```python
from build123d import *

# Parameters (mm, degrees)
SCHIZZO1_R                   = 20
SCHIZZO1_R_2                 = 1.6
ESTRUSIONE_ESTRUSIONE1_DEPTH = 10
TAGLIO_ESTRUSIONE1_DEPTH     = 3
RACCORDO1_R                  = 2
SCHIZZO3_R                   = 5
SCHIZZO3_R_2                 = 1.6
ESTRUSIONE_ESTRUSIONE2_DEPTH = 0.5


with BuildPart() as part:
    # Schizzo1 → Estrusione-Estrusione1 (new body)
    with BuildSketch(Plane.XY):
        Circle(SCHIZZO1_R)
        Circle(SCHIZZO1_R_2, mode=Mode.SUBTRACT)
    extrude(amount=ESTRUSIONE_ESTRUSIONE1_DEPTH)

    # Schizzo2 → Taglio-Estrusione1 (cut)
    with BuildSketch(Plane.XY.offset(10)):
        Polygon((3.175426481, 0), (1.58771324, 2.75), (-1.58771324, 2.75), (-3.175426481, 0), (-1.58771324, -2.75), (1.58771324, -2.75), align=None)
    extrude(amount=-TAGLIO_ESTRUSIONE1_DEPTH, mode=Mode.SUBTRACT)

    # Raccordo1
    raccordo1_edges = [part.edges().sort_by_distance(p)[0] for p in [
        (-20, 0, 0),
        (-20, 0, 10),
    ]]
    fillet(raccordo1_edges, radius=RACCORDO1_R)

    # Schizzo3 → Estrusione-Estrusione2 (add)
    with BuildSketch(Plane(origin=(0, 0, 0), x_dir=(-1, 0, 0), z_dir=(0, 0, -1))):
        Circle(SCHIZZO3_R)
        Circle(SCHIZZO3_R_2, mode=Mode.SUBTRACT)
    extrude(amount=ESTRUSIONE_ESTRUSIONE2_DEPTH)


solid = part.part
```
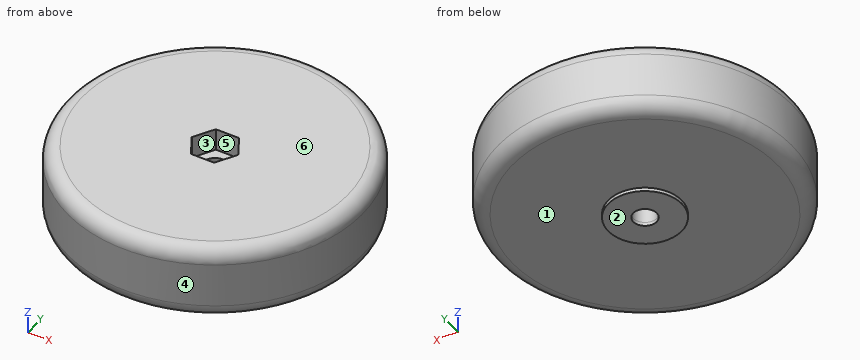
Geometry check sheet. Reference: the model listing, model coordinates, mm. Face numbers are marked on the shaded views. A direction names the side the tool comes from. Coordinates: 2 decimals unless noted, no trailing zeros. Write each loop counter-clockwise with the first axis right and the second up, starting at its lowest first coordinate (ties: lowest second). Pieces come first, ordered by that corner, then holes. Notation, with made-up numbers: M -7.75,48.5 L 35.25,48.5 A31 ccw 35.25,76.5 Z; hole C 60,-39.5 d11. An arc over 180 degrees is marked long. Use one line per item in the form item = value. Start each with the question number.
1) Set-up check for the marked faces 1, 2 and 3: record each of +Z, -Z, +X, -X, +Y, -Y from which the full face is reachable in a straight line by a thin tool's end or side.
2) Release check for a two-part mould opening along X. For the marked faces 4, 5 and 6 record: pulls with the +X half, pulls with the -X half, needs draft (parallel to the pull), parting line crosses it, or undercut.
3) Go/stop test with flat-tipped pins: pin 1 Ø1.6 at (x, y) = (1, -0.5) entering from +Z; pin 2 Ø1.5 at (x, z) = (-0.5, 9) entering from +Y; pin 3 Ø2.5 at (x, y) = (0, 0) entering from +Z; pin 4 Ø1.5 at (x, z) = (0.5, 2.5) entering from -Y. Record where each tip stops, or that it passes through.
4) Section check A-A on x = 0. Enter the section's corners in (y, z), and give its area (3 significant figures).
5) Thickness scan on probe 1 along Y at (x, z) = (0, 5.75); probe 2 along Z at (x, y) = (-4, -8); probe 3 along Y at (x, z) = (0, -0.4). Record the ranges inside material, lowest first. Write a range as from..to.
Responses:
q1.face_1 = -Z
q1.face_2 = -Z, +X, -X, +Y, -Y
q1.face_3 = +Z
q2.face_4 = parting line crosses it
q2.face_5 = undercut
q2.face_6 = needs draft
q3.pin_1 = 7
q3.pin_2 = 19.98
q3.pin_3 = through
q3.pin_4 = -20
q4.outline = M -20,2 A2 ccw -18,0 L -5,0 L -5,-0.5 L -1.6,-0.5 L -1.6,7 L -2.75,7 L -2.75,10 L -18,10 A2 ccw -20,8 Z; M 1.6,-0.5 L 5,-0.5 L 5,0 L 18,0 A2 ccw 20,2 L 20,8 A2 ccw 18,10 L 2.75,10 L 2.75,7 L 1.6,7 Z
q4.area = 361 mm2
q5.probe_1 = -20..-1.6, 1.6..20
q5.probe_2 = 0..10
q5.probe_3 = -5..-1.6, 1.6..5
